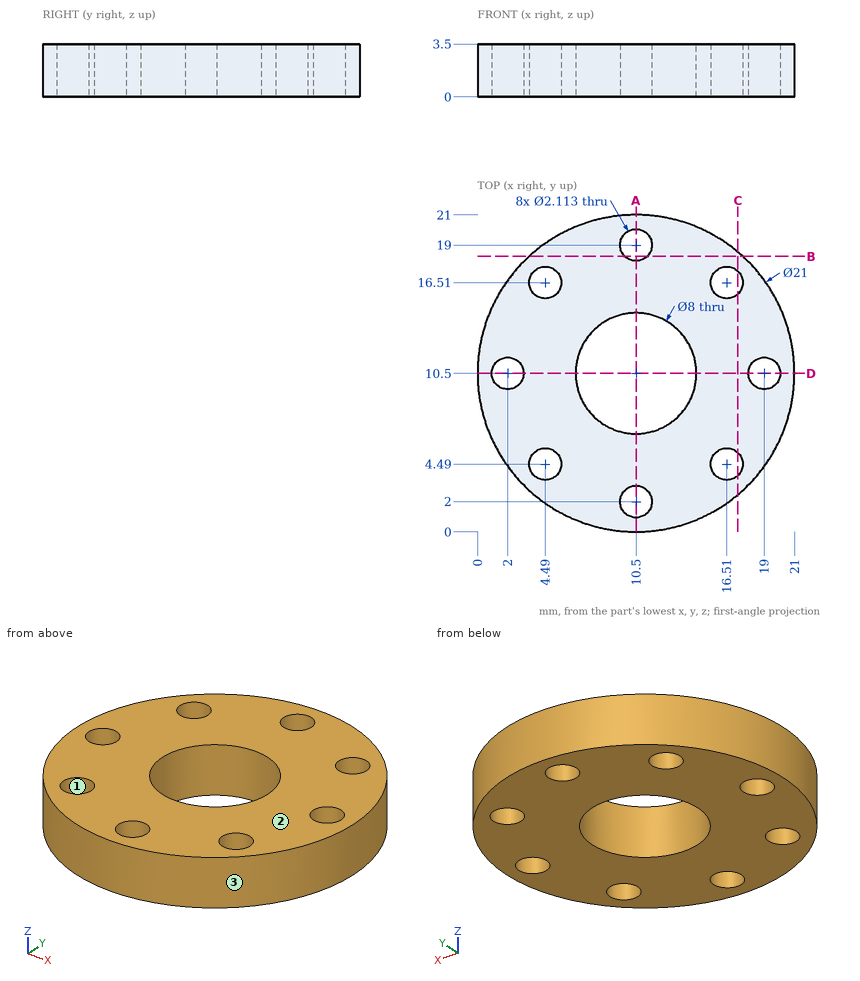
Geometry check sheet. Reference: drawing and pictorial views, mm from the part's lowest x, y, z. Coordinates: 2 decimals unless noted, no trailing zeros. Write each loop counter-clockwise with the first axis right and the second up, starting at its lowest first coordinate (ties: lowest second). Pieces come first, ordered by that corner, then holes. Notation, with made-up numbers: M 61,75.5 L 71,75.5 A14 ccw 71,93.5 Z; hole C 82.25,-34.5 d9. An arc over 180 degrees is marked long. Write item = value, one per line. Start each with the question number.
1. Sectioned sample at C-C (x = 17.25). Record the cut outline in (y, z) (1 decimal).
2. Sectioned sample at A-A (x = 10.5). Record the cut outline in (y, z).
3. Go/stop test with flat-tipped pins: pin 1 (1.5 mm diameter, centred on y = 8.5, z = 2.5, fed in from -X) (1 decimal); pin 2 (2.5 mm diameter, centred on x = 16.51, y = 4.49, fed in from -Z); pin 3 (1.5 mm diameter, centred on x = 3.5, z = 3, fed in from -Y); pin 4 (2 mm diameter, centred on x = 13, z = 1, fed in from -Y). Record where each tip stops, or that it passes through.
4. Sectioned sample at B-B (y = 18.25). Record the cut outline in (x, z) (1 decimal).
5. Mould release check, pull along Y, two halves, no side actions. Record for the marked faces 1, 2 and 3: pulls with the +Y half, pulls with the -Y half, needs draft (parallel to the pull), parting line crosses it, or undercut.
6. Thickness scan on probe 1 along Y at (x, z) = (10.5, 1); probe 2 along X at (y, z) = (10.25, 1.2); probe 3 along X at (y, z) = (17.25, 2.75) (1 decimal). Record the ranges inside material, lowest first.
The answers:
q1.outline = M 2.5,0 L 3.7,0 L 3.7,3.5 L 2.5,3.5 Z; M 5.2,0 L 15.8,0 L 15.8,3.5 L 5.2,3.5 Z; M 17.3,0 L 18.5,0 L 18.5,3.5 L 17.3,3.5 Z
q2.outline = M 0,0 L 0.94,0 L 0.94,3.5 L 0,3.5 Z; M 3.06,0 L 6.5,0 L 6.5,3.5 L 3.06,3.5 Z; M 14.5,0 L 17.94,0 L 17.94,3.5 L 14.5,3.5 Z; M 20.06,0 L 21,0 L 21,3.5 L 20.06,3.5 Z
q3.pin_1 = 0.1
q3.pin_2 = 0
q3.pin_3 = 2.06
q3.pin_4 = 0.11
q4.outline = M 3.4,0 L 9.8,0 L 9.8,3.5 L 3.4,3.5 Z; M 11.2,0 L 17.6,0 L 17.6,3.5 L 11.2,3.5 Z
q5.face_1 = undercut
q5.face_2 = needs draft
q5.face_3 = parting line crosses it
q6.probe_1 = 0 to 0.94, 3.06 to 6.5, 14.5 to 17.94, 20.06 to 21
q6.probe_2 = 0 to 0.97, 3.03 to 6.51, 14.49 to 17.97, 20.03 to 21
q6.probe_3 = 2.5 to 3.7, 5.2 to 15.8, 17.3 to 18.5
